For this review, take the finished solid that the model builds, in its own axes (mm). A direction names the side the tool comes from. Give positions to 0.01 mm unless a question says otherwise; leave off trailing zeros. Loops run counter-clockwise (first coordinate to the right, second up) from the corner with the lowest first, then second, coordinate; pieces in that order, holes last. Notation, with made-up numbers: (66, 15) - (80, 15) arc R7 cw to (80, 22) - close; hole circle Ø5 at (73.25, 56.25). An arc over 180 degrees is marked (long way). Use CSV: the item, a comma, the result in double quotes. Start each with the question number.
1. Take a section at A-A on z = 2.25. Give the boundary of the cut face in (x, y), plus the area to 3 significant figures.
2. Wall thickness on line 1 (Z direction, x = 8, y = -8.75); line 2 (Y direction, x = -3.5, z = 1.45); line 3 (Y direction, x = -0.25, z = 1.55): over which ranges is each line inside the solid? List them lowest first.
3. Take a section at C-C on z = 0.5. Give the boundary of the cut face in (x, y).
4. For pin 1 (13.5 mm diameter, centred on x = -2.5, y = -6.5, fed in from +Z); pin 2 (2 mm diameter, centred on x = -9.5, z = 2.5, fed in from +Y); pin 3 (1.5 mm diameter, centred on y = 8.5, z = 3, fed in from -X); pin 4 (1.4 mm diameter, centred on x = 11, z = 2.5, fed in from +Y), all flat-tipped, find the tip position at first contact; note any pin that passes through.
5. Take a section at B-B on y = -6.5. Give the boundary of the cut face in (x, z).
6. For faces 1 (the cylindrical face through (-2.11, 11.63, 1.23)), 2 (the cylindrical face through (2.146, -11.598, 1.252)), 3 (the flat face through (12, 0, 2)), 4 (the flat face through (-12, 0, 2)), 5 (the flat face through (-11, 2, 3.7)), list the 3-axis set-ups (+Z, -Z, +X, -X, +Y, -Y) from which the entire face can be reached by the end or side of a thin tool; tool diameter is ignored.
```python
from build123d import *

# Parameters (mm, degrees)
BOSS_EXTRUDE1_DEPTH = 1.7
FILLET1_R           = 3
BOSS_EXTRUDE2_DEPTH = 2
FILLET2_R           = 0.5


with BuildPart() as part:
    # Sketch1 → Boss-Extrude1 (new body)
    with BuildSketch(Plane.XY):
        with BuildLine():
            ThreePointArc((-11, 0), (-8.110050705, 7.431492284), (-0.95871317, 10.958141679))
            Line((-0.95871317, 10.958141679), (-1.119951294, 12.80110187))
            ThreePointArc((-1.119951294, 12.80110187), (-9.474013778, 8.681334168), (-12.85, 0))
            Line((-12.85, 0), (-11, 0))
        make_face()
        with BuildLine():
            ThreePointArc((-10, 0), (-7.372773368, 6.755902076), (-0.871557427, 9.961946981))
            Line((-0.871557427, 9.961946981), (-0.95871317, 10.958141679))
            ThreePointArc((-0.95871317, 10.958141679), (-8.110050705, 7.431492284), (-11, 0))
            Line((-11, 0), (-10, 0))
        make_face()
        with BuildLine():
            Line((-0.95871317, 10.958141679), (-0.871557427, 9.961946981))
            ThreePointArc((-0.871557427, 9.961946981), (6.755902076, 7.372773368), (10, 0))
            Line((10, 0), (11, 0))
            ThreePointArc((11, 0), (7.431492284, 8.110050705), (-0.95871317, 10.958141679))
        make_face()
        with BuildLine():
            ThreePointArc((10, 0), (7.372773368, -6.755902076), (0.871557427, -9.961946981))
            Line((0.871557427, -9.961946981), (0.95871317, -10.958141679))
            ThreePointArc((0.95871317, -10.958141679), (8.110050705, -7.431492284), (11, 0))
            Line((11, 0), (10, 0))
        make_face()
        with BuildLine():
            Line((0.95871317, -10.958141679), (0.871557427, -9.961946981))
            ThreePointArc((0.871557427, -9.961946981), (-6.755902076, -7.372773368), (-10, 0))
            Line((-10, 0), (-11, 0))
            ThreePointArc((-11, 0), (-7.431492284, -8.110050705), (0.95871317, -10.958141679))
        make_face()
        with BuildLine():
            ThreePointArc((11, 0), (8.110050705, -7.431492284), (0.95871317, -10.958141679))
            Line((0.95871317, -10.958141679), (1.119951294, -12.80110187))
            ThreePointArc((1.119951294, -12.80110187), (9.474013778, -8.681334168), (12.85, 0))
            Line((12.85, 0), (11, 0))
        make_face()
    extrude(amount=BOSS_EXTRUDE1_DEPTH)

    # Fillet1
    # the kernel refuses this fillet: 3 mm, written as the material it takes off along each edge
    with BuildSketch(Plane(origin=(0.369605462, -4.22460976, 1.7), x_dir=(0.9961946980917454, 0.08715574274765832, 0), z_dir=(0.08715574274765833, -0.9961946980917455, 0))) as fillet1_piece_1_section:
        with BuildLine():
            CenterArc((2.703701167, -3), FILLET1_R, 90, 64.320711381)
            Line((0, -1.7), (0, 0))
            Line((0, 0), (2.703701167, 0))
        make_face()
    fillet1_piece_1 = extrude(amount=15.368505835, mode=Mode.PRIVATE)
    fillet1_piece_1 = fillet1_piece_1 - Plane(origin=(0, 0, 1.24476439), x_dir=(1, 0, 0), z_dir=(0, 0, -1)) * Cylinder(11, 42, mode=Mode.PRIVATE)
    add(fillet1_piece_1, mode=Mode.SUBTRACT)
    with BuildSketch(Plane(origin=(-1.709059003, 19.53463379, 1.7), x_dir=(0, 0, -1), z_dir=(0.08715574274761673, -0.9961946980917492, 0))) as fillet1_piece_2_section:
        with BuildLine():
            CenterArc((3, -2.703701167), FILLET1_R, 115.679288619, 64.320711381)
            Line((0, -2.703701167), (0, 0))
            Line((0, 0), (1.7, 0))
        make_face()
    fillet1_piece_2 = extrude(amount=15.368505835, mode=Mode.PRIVATE)
    fillet1_piece_2 = fillet1_piece_2 - Plane(origin=(0, 0, 1.24476439), x_dir=(1, 0, 0), z_dir=(0, 0, -1)) * Cylinder(11, 42, mode=Mode.PRIVATE)
    add(fillet1_piece_2, mode=Mode.SUBTRACT)

    # Sketch2 → Boss-Extrude2 (add)
    with BuildSketch(Plane.XY.offset(1.7)):
        with BuildLine():
            Line((-12.85, 0), (-11, 0))
            Line((-11, 0), (-10, 0))
            ThreePointArc((-10, 0), (-9.84807753, 1.736481777), (-9.396926208, 3.420201433))
            Line((-9.396926208, 3.420201433), (-12.075050177, 4.394958842))
            ThreePointArc((-12.075050177, 4.394958842), (-12.654779626, 2.231379083), (-12.85, 0))
        make_face()
        with BuildLine():
            ThreePointArc((10, 0), (9.84807753, -1.736481777), (9.396926208, -3.420201433))
            Line((9.396926208, -3.420201433), (12.075050177, -4.394958842))
            ThreePointArc((12.075050177, -4.394958842), (12.654779626, -2.231379083), (12.85, 0))
            Line((12.85, 0), (11, 0))
            Line((11, 0), (10, 0))
        make_face()
    extrude(amount=BOSS_EXTRUDE2_DEPTH)

    # Fillet2
    fillet2_edges = [part.edges().sort_by_distance(p)[0] for p in [
        (-9.84807753, 1.736481777, 3.7),
        (-10.735988192, 3.907580137, 3.7),
        (-12.654779626, 2.231379083, 3.7),
        (-11.425, 0, 3.7),
        (9.84807753, -1.736481777, 3.7),
        (10.735988192, -3.907580137, 3.7),
        (12.654779626, -2.231379083, 3.7),
        (11.425, 0, 3.7),
    ]]
    fillet(fillet2_edges, radius=FILLET2_R)


solid = part.part
```
Check result:
1,outline,"(-12.85, 0) - (-10, 0) arc R10 cw to (-9.4, 3.42) - (-12.08, 4.39) arc R12.85 ccw to start; (9.4, -3.42) - (12.08, -4.39) arc R12.85 ccw to (12.85, 0) - (10, 0) arc R10 cw to start"
1,area,"22.7 mm²"
2,line 1,"z = 0 to 1.7"
2,line 2,"y = -10.43 to -9.37, 9.37 to 12.36"
2,line 3,"y = -11 to -10, 10 to 11"
3,outline,"(-12.85, 0) - (-11, 0) arc R11 ccw to (1.26, -10.93) - (1.42, -12.77) arc R12.85 ccw to (12.85, 0) - (11, 0) arc R11 ccw to (-1.26, 10.93) - (-1.42, 12.77) arc R12.85 ccw to start; hole circle Ø20 at (0, 0)"
4,pin 1,"stops at z = 1.7"
4,pin 2,"stops at y = 9.27"
4,pin 3,"passes through"
4,pin 4,"stops at y = 0"
5,outline,"(-8.87, 0) - (-7.6, 0) - (-7.6, 1.7) - (-8.87, 1.7) - close; (7.6, 0) - (11.08, 0) - (11.08, 1.7) - (7.6, 1.7) - close"
6,face 1,"+Z, +Y"
6,face 2,"+Z, -Y"
6,face 3,"+Z, +X, +Y"
6,face 4,"+Z, -X, -Y"
6,face 5,"+Z, +X, -X, +Y, -Y"
